Verification items for the finished model (mm, model axes). A direction names the side the tool comes from. Give positions to 0.01 mm unless a question says otherwise; leave off trailing zeros. Write each loop counter-clockwise with the first axis right and the second up, starting at its lowest first coordinate (ties: lowest second). Pieces come first, ordered by that corner, then holes. Notation, with made-up numbers: M 47,26.25 L 78,26.25 A12 cw 78,43.25 Z; hole C 24.25,54 d8. An arc over 180 degrees is marked long. Write item = value, one per line.
from build123d import *

# Parameters (mm, degrees)
CYLINDER001_R     = 0.5
CYLINDER001_DEPTH = 4
ARRAY001_Y_COUNT  = 2
ARRAY001_Y_PITCH  = 21
ARRAY001_Z_COUNT  = 4
ARRAY001_Z_PITCH  = 6
BOX001_W          = 4
BOX001_H          = 21
BOX001_DEPTH      = 74
BOX_W             = 4
BOX_H             = 40
BOX_DEPTH         = 36
FILLET001_R       = 6
FILLET004_R       = 1
CYLINDER_R        = 2
CYLINDER_DEPTH    = 4
ARRAY_Y_COUNT     = 2
ARRAY_Y_PITCH     = 21
ARRAY_Z_COUNT     = 4
ARRAY_Z_PITCH     = 6


with BuildPart() as camera_hole_array:
    # Cylinder001 → Cylinder001 (new body)
    with BuildSketch(Plane(origin=(0, 0, 0), x_dir=(0, 0, -1), z_dir=(1, 0, 0))):
        Circle(CYLINDER001_R)
    extrude(amount=CYLINDER001_DEPTH)

    # Array001 Y: camera hole array ×2


with BuildPart() as camera_hole_array_1:
    add(camera_hole_array.part)
    with Locations(*[(0, i * ARRAY001_Y_PITCH, 0) for i in range(1, ARRAY001_Y_COUNT)]):
        add(camera_hole_array.part)

    # Array001 Z: camera hole array ×4


with BuildPart() as camera_hole_array_2:
    add(camera_hole_array_1.part)
    with Locations(*[(0, 0, i * ARRAY001_Z_PITCH) for i in range(1, ARRAY001_Z_COUNT)]):
        add(camera_hole_array_1.part)


with BuildPart() as camera_hole_array_3:
    # Array001 placement: moved
    add(camera_hole_array_2.part.moved(Location((0, 7, 2))))


with BuildPart() as camera_plate_hole:
    # Box001 → Box001 (new body)
    with BuildSketch(Plane(origin=(0, 7, -4), x_dir=(1, 0, 0), z_dir=(0, 0, 1))):
        with Locations((2, 10.5)):
            Rectangle(BOX001_W, BOX001_H)
    extrude(amount=BOX001_DEPTH)


with BuildPart() as camera_plate_cut_fillet:
    # Box → Box (new body)
    with BuildSketch(Plane(origin=(0, -2.5, -11), x_dir=(1, 0, 0), z_dir=(0, 0, 1))):
        with Locations((2, 20)):
            Rectangle(BOX_W, BOX_H)
    extrude(amount=BOX_DEPTH)

    # Fillet001
    fillet001_edges = [camera_plate_cut_fillet.edges().sort_by_distance(p)[0] for p in [
        (2, -2.5, 25),
        (2, 37.5, 25),
    ]]
    fillet(fillet001_edges, radius=FILLET001_R)

    # Cut001: cut camera plate hole
    add(camera_plate_hole.part, mode=Mode.SUBTRACT)

    # Fillet004
    fillet004_edges = [camera_plate_cut_fillet.edges().sort_by_distance(p)[0] for p in [
        (2, 7, 25),
        (2, 28, 25),
    ]]
    fillet(fillet004_edges, radius=FILLET004_R)


with BuildPart() as camera_holder_cut:
    # Cylinder → Cylinder (new body)
    with BuildSketch(Plane(origin=(0, 0, 0), x_dir=(0, 0, -1), z_dir=(1, 0, 0))):
        Circle(CYLINDER_R)
    extrude(amount=CYLINDER_DEPTH)

    # Array Y: camera holder cut ×2


with BuildPart() as camera_holder_cut_1:
    add(camera_holder_cut.part)
    with Locations(*[(0, i * ARRAY_Y_PITCH, 0) for i in range(1, ARRAY_Y_COUNT)]):
        add(camera_holder_cut.part)

    # Array Z: camera holder cut ×4


with BuildPart() as camera_holder_cut_2:
    add(camera_holder_cut_1.part)
    with Locations(*[(0, 0, i * ARRAY_Z_PITCH) for i in range(1, ARRAY_Z_COUNT)]):
        add(camera_holder_cut_1.part)


with BuildPart() as camera_holder_cut_3:
    # Array placement: moved
    add(camera_holder_cut_2.part.moved(Location((0, 7, 2))))

    # Fusion: union camera plate cut fillet
    add(camera_plate_cut_fillet.part)

    # Cut: cut camera hole array
    add(camera_hole_array_3.part, mode=Mode.SUBTRACT)


with BuildPart() as camera_holder_cut_4:
    # Cut placement: moved
    add(camera_holder_cut_3.part.moved(Location((-10, 11, 11))))


solid = camera_holder_cut_4.part
1) Cross-section at C-C on z = 11.5. Record the boundary of the cut face in (x, y), plus the area to 3 significant figures.
From the geometry:
outline = M -10,8.5 L -6,8.5 L -6,19.32 L -10,19.32 Z; M -10,37.68 L -6,37.68 L -6,48.5 L -10,48.5 Z
area = 86.6 mm^2
2) Cross-section at D-D on x = -8.25. Count the separate pieces of the cut face and the enclosed holes in it, plus the area to 3 significant figures.
From the geometry:
separate_pieces = 1
enclosed_holes = 8
area = 859 mm^2
3) Depth check by flat-ended pin: P1, Ø1.6, axis at x = -9, z = 33.5, coming from the -Y side; P2, Ø2, axis at x = -8, z = 34.5, coming from the +Y side; P3, Ø2, axis at x = -8, y = 37.5, coming from the +Z side. Enter the tip coordinate at first touch or a pass-through.
From the geometry:
P1 = 9.14
P2 = 47.37
P3 = 32.94
4) Material ranges on probe 1 along Y at (x, z) = (-7.5, 19); probe 2 along Y at (x, z) = (-6.2, 16); probe 3 along Z at (x, y) = (-7.1, 38), recorded low to high. Write a range as from..to.
From the geometry:
probe_1 = 8.5..17.5, 18.5..20, 37..38.5, 39.5..48.5
probe_2 = 8.5..18, 39..48.5
probe_3 = 0..7, 11.27..14.73, 17.27..20.73, 23.27..26.73, 29.27..32.73
5) Cross-section at B-B on y = 37.5. Record the boundary of the cut face in (x, z).
From the geometry:
outline = M -10,0 L -6,0 L -6,7 L -10,7 Z; M -10,11.68 L -6,11.68 L -6,14.32 L -10,14.32 Z; M -10,17.68 L -6,17.68 L -6,20.32 L -10,20.32 Z; M -10,23.68 L -6,23.68 L -6,26.32 L -10,26.32 Z; M -10,29.68 L -6,29.68 L -6,32.32 L -10,32.32 Z
6) Tool access check on faces 5 (the cylindrical face through (-8, 37, 25)), 6 (the cylindrical face through (-8.028, 39.301, 35.715)), 7 (the flat face through (-6, 19, 14)). Record the directions out of +Z, -Z, +X, -X, +Y, -Y that give a thin tool (end or side, any length) a straight path to the whole face; none if there is none.
From the geometry:
face_5 = +X, -X
face_6 = +Z, +X, -X
face_7 = +Z, -Z, +X, +Y, -Y
7) Cross-section at A-A on z = 19. Record the boundary of the cut face in (x, y).
From the geometry:
outline = M -10,8.5 L -6,8.5 L -6,17.5 L -10,17.5 Z; M -10,18.5 L -6,18.5 L -6,20 L -10,20 Z; M -10,37 L -6,37 L -6,38.5 L -10,38.5 Z; M -10,39.5 L -6,39.5 L -6,48.5 L -10,48.5 Z
8) Draft check along Z on faces 1 (the flat face through (-8, 8.5, 15)), 2 (the cylindrical face through (-8.028, 18.496, 13.065)), 3 (the flat face through (-8, 29, 0)), 4 (the flat face through (-8, 16, 36)). Enter one of: +Z half, -Z half, draft (parallel to the pull), parting line (faces both ways), or undercut.
From the geometry:
face_1 = draft
face_2 = undercut
face_3 = -Z half
face_4 = +Z half
